Autodesk Inventor part; units mm, degrees
ref_plane "Work Plane1" through (104.775, 0, 0) normal (0, 0, -1) x (1, 0, 0)
ref_plane "YZ Plane" through (0, 0, 0) normal (1, 0, 0) x (0, 1, 0)
ref_plane "XZ Plane" through (0, 0, 0) normal (0, 1, 0) x (-1, 0, 0)
sketch "Sketch1" plane through (0, 0, 0) normal (0, 0, 1) x (1, 0, 0)
  line L0 (25, 0) -> (25, 3)
  line L1 (25, 3) -> (7, 3)
  line L2 (7, 3) -> (6.3865, 3)
  line L3 (0, 5.67) -> (0, 2.3094)
  line L4 (0, 2.3094) -> (2.67, 2.3094)
  line L5 (2.67, 2.3094) -> (4.0033, 0)
  line L6 (4.0033, 0) -> (25, 0)
  line L7 (0, 5.67) -> (1.05, 5.67)
  line L8 (1.05, 5.67) -> (3.72, 3)
  line L9 (6.3865, 3) -> (3.72, 3)
  line L10 (7, 3) -> (3.72, 3) construction
  line L11 (3.72, 3) -> (3.72, 3)
  line L12 (-5, 0) -> (30, 0)
  line L13 (0, -1.134) -> (0, 6.804)
  dimension "d0" = 25
  dimension "d1" = 18
  dimension "d2" = 2.67
  dimension "d3" = 6
  dimension "d6" = 3.72
  dimension "d7" = 45
  dimension "d8" = 4.6188
  dimension "d9" = 60
  dimension "d10" = 11.34
  dimension "d11" = 6
  dimension "d12" = 0.6135
revolve "Body" add sketch "Sketch1" angle 360 about axis through (4.0033, 0, 0) along (1, 0, 0) contours L6 L5 L4 L3 L7 L8 L9 L2 L1 L0
sketch "Sketch2" plane through (0, 0, 0) normal (-1, 0, 0) x (0, 0, 1)
  circle A0 centre (0, 0) radius 2.3094
  line L0 (0, -7.938) -> (0, 7.938)
  line L1 (-7.938, 0) -> (7.938, 0)
  line L2 (2.3094, 0) -> (1.1547, -2)
  line L3 (1.1547, -2) -> (-1.1547, -2)
  line L4 (-1.1547, -2) -> (-2.3094, 0)
  line L5 (-2.3094, 0) -> (-1.1547, 2)
  line L6 (-1.1547, 2) -> (1.1547, 2)
  line L7 (1.1547, 2) -> (2.3094, 0)
  point P0 (0, 2.3094)
extrude "Slot" add sketch "Sketch2" against normal up to next contours L7 A0 | A0 L2 | L6 L0 A0 | A0 L0 L3 | L0 L6 A0 | A0 L3 L0 | L4 A0 | A0 L5
thread "Thread"
chamfer "Chamfer1" distance 0.6135 distance2 0.6135 1 edges at (25, -3, 0) measured on face at (25, -0.1411, -0.823)
ref_plane "Work Plane1" through (104.775, 0, 0) normal (0, 0, -1) x (1, 0, 0)
equation "\"d15\" = GEL"
equation "\"d17\" = -0.5 * SPD + 0.5 * GD"
equation "\"d18\" = GUL"
equation "\"d0\" = NLG"
equation "\"d1\" = GEL"
equation "\"d2\" = INTI"
equation "\"d3\" = GD"
equation "\"d6\" = KOH"
equation "\"d7\" = 0.5 * SEWI"
equation "\"d8\" = 1.1547 * SW"
equation "\"d10\" = KOD"
equation "\"d11\" = BDM"
equation "\"d12\" = GAL"
equation "\"NLG\" = 25"
equation "\"INTI\" = 2.67"
equation "\"GEL\" = 18"
equation "\"GAL\" = 0.61345 * PTC"
equation "\"KOH\" = 3.72"
equation "\"KOD\" = 11.34"
equation "\"GUL\" = 0.61345 * PTC"
equation "\"SPD\" = NND - 1.2269 * PTC"
equation "\"BDM\" = NND"
equation "\"GD\" = NND"
equation "\"SEWI\" = 90deg"
equation "\"SW\" = 4"
equation "\"TOA\" = 30deg"
equation "\"GD1\" = THREADDIA - 1.2269 * PTC"
equation "\"EPV\" = 6.72"
equation "\"THREADDIA\" = 6"
equation "\"PTC\" = 1"
equation "\"NND\" = 6"
equation "\"E0\" = 4.62"
equation "\"THREADDESC\" = 1.2345"
properties part number "ISO 10642 - M6 x  25" material "Steel"
Check sheet for the modelled part. Datum: model origin and axes. Units: mm. A direction names the side the tool comes from. Coordinates: 2 decimals unless noted, no trailing zeros. Write each loop counter-clockwise with the first axis right and the second up, starting at its lowest first coordinate (ties: lowest second). Pieces come first, ordered by that corner, then holes. Notation, with made-up numbers: M 28.25,-20.75 L 36.25,-20.75 A13 cw 36.25,-12.75 Z; hole C 53,-30 d9. An arc over 180 degrees is marked long. Use one line per item in the form item = value.
Item 1: Release check for a two-part mould opening along Y. For faces 3 (the face through (14, -3, 0)), 4 (the face through (0, 0.08, 2.44)), 5 (the face through (1.404, 1.014, 1.724)) record: pulls with the +Y half, pulls with the -Y half, needs draft (parallel to the pull), parting line crosses it, or undercut.
Answer below:
face_3 = parting line crosses it
face_4 = needs draft
face_5 = undercut
Item 2: Gauge pin test, flat ends, axial feed: pin 1 Ø5 at (x, y) = (11.5, -2) entering from +Z; pin 2 Ø5 at (x, y) = (12.5, -3.5) entering from +Z; pin 3 Ø1.5 at (x, z) = (21, -1) entering from +Y; pin 4 Ø1.5 at (x, z) = (15, 4.5) entering from +Y. Record the tip position at first contact, or that the pin passes through.
Answer below:
pin_1 = 3
pin_2 = 2.83
pin_3 = 2.99
pin_4 = through
Item 3: Set-up check for faces 1 (the face through (1.404, -1.014, -1.724)), 2 (the face through (3.553, 1.461, 2.81)): record each of +Z, -Z, +X, -X, +Y, -Y from which the full face is reachable in a straight line by a thin tool's end or side.
Answer below:
face_1 = -X
face_2 = +X
Item 4: Sectioned sample at A-A, the plane x = 7. Record the cut outline in (y, z).
Answer below:
outline = C 0,0 d6
Item 5: Material ranges on L1, parallel to Y at x = 17, z = -1.5; L2, parallel to Z at x = 7.75, y = -0.5; L3, parallel to Y at x = 2.5, z = 0, recorded low to high. Write a range as from..to.
Answer below:
L1 = -2.6..2.6
L2 = -2.96..2.96
L3 = -4.22..-2, 2..4.22
